Part model, mm, in its own coordinate system. A direction names the side the tool comes from. Give positions to 0.01 mm unless a question says otherwise; leave off trailing zeros. Order: outer loops, then holes, each group sorted by start corner. A loop starts at its lowest first (then second) coordinate and runs counter-clockwise, first axis right, second up. Notation, with made-up numbers: M -23.75,67 L 33.25,67 A35 cw 33.25,100 Z; hole C 22,51 d8. An arc over 180 degrees is marked long. Answer as a JSON object with one key per item and string values.
from build123d import *

# Parameters (mm, degrees)
F1_DEPTH = 10
F2_R     = 5
F3_R     = 2.5
F4_R     = 1.5
F5_DEPTH = 25


with BuildPart() as f1:
    # F0 (on Front) → F1 (new body)
    with BuildSketch(Plane.XZ):
        Polygon((-40.5, 0), (0, 0), (0, -6.2), (7, -6.2), (7, 7.8), (-123, 22.8), (-143, 22.8), (-143, 12.8), (-118, 12.8), (-40.5, -13.2), (-34.5, -13.2), (-34.5, -6.2), (-40.5, -6.2), align=None)
    extrude(amount=F1_DEPTH)

    # F2
    f2_edges = [f1.edges().sort_by_distance(p)[0] for p in [
        (7, -5, 7.8),
    ]]
    fillet(f2_edges, radius=F2_R)

    # F3
    f3_edges = [f1.edges().sort_by_distance(p)[0] for p in [
        (-34.5, -5, -13.2),
        (-40.5, -5, -13.2),
    ]]
    fillet(f3_edges, radius=F3_R)

    # F4 (on face) → F5 (cut)
    with BuildSketch(Plane.XY.offset(22.8)):
        with Locations((-128, -5)):
            Circle(F4_R)
        with Locations((-138, -5)):
            Circle(F4_R)
    extrude(amount=-F5_DEPTH, mode=Mode.SUBTRACT)


solid = f1.part
1. Which spindle directions (+Z, -Z, +X, -X, +Y, -Y) get a long thin tool onto all of the face, cutting with end or side? Do faces 1 (the flat face through (0, -5, -3)), 2 (the flat face through (-131, -5, 12.8)), 3 (the flat face through (-34.5, -5, -8)). Say none if no direction does.
Worked answers:
{"face 1": "-Z, +Y, -Y", "face 2": "-Z, -X, +Y, -Y", "face 3": "-Z, +X, +Y, -Y"}
2. Pin check, flat tips, straight feed: P1, Ø3.5, axis at x = 3.5, y = -5, coming from the -Z side; P2, Ø1.8, axis at x = -39, y = -3, coming from the +Z side; P3, Ø5, axis at y = -6, z = -9, coming from the +X side; P4, Ø2.5, axis at x = -138, y = -5, coming from the -Z side. Stop position of each tip, or through.
Worked answers:
{"P1": "stops at z = -6.2", "P2": "stops at z = 13.21", "P3": "stops at x = -34.5", "P4": "passes through"}
3. Cut at B-B on y = -5. Give the cut face in (x, z).
Worked answers:
{"outline": "M -143,12.8 L -139.5,12.8 L -139.5,22.8 L -143,22.8 Z; M -136.5,12.8 L -129.5,12.8 L -129.5,22.8 L -136.5,22.8 Z; M -126.5,12.8 L -118,12.8 L -40.89,-13.07 A2.5 ccw -40.09,-13.2 L -37,-13.2 A2.5 ccw -34.5,-10.7 L -34.5,-6.2 L -40.5,-6.2 L -40.5,0 L 0,0 L 0,-6.2 L 7,-6.2 L 7,3.34 A5 ccw 2.57,8.31 L -123,22.8 L -126.5,22.8 Z"}
4. Two-plate mould, pull along X, no slides. Class faces 4 (the flat face through (-79.983, -4.93, 0.046)), 5 (the flat face through (-133, -5, 22.8)), 6 (the cylindrical face through (-139.5, -4.93, 17.87)): +X half, -X half, draft (parallel to the pull), parting line (faces both ways), or undercut.
Worked answers:
{"face 4": "-X half", "face 5": "draft", "face 6": "undercut"}
5. Probe line 1 along Y through (x, z) = (-138, 19); line 2 along Z through (x, y) = (-126.5, -2); line 3 along Z through (x, y) = (-52.5, -5.5). List the from-to ranges inside material, lowest first.
Worked answers:
{"line 1": "y = -10 to -6.5, -3.5 to 0", "line 2": "z = 12.8 to 22.8", "line 3": "z = -9.17 to 14.67"}
6. Cut at C-C on z = 18. Give the cut face in (x, y), plus the area to 3 significant figures.
Worked answers:
{"outline": "M -143,-10 L -81.4,-10 L -81.4,0 L -143,0 Z; hole C -138,-5 d3; hole C -128,-5 d3", "area": "602 mm^2"}
7. Cut at D-D on z = -2. Give the cut face in (x, y).
Worked answers:
{"outline": "M -73.88,-10 L -40.5,-10 L -40.5,0 L -73.88,0 Z; M 0,-10 L 7,-10 L 7,0 L 0,0 Z"}
8. Cut at A-A on x = -38.5. Give the cut face in (y, z), plus the area to 4 significant figures.
Worked answers:
{"outline": "M -10,-13.2 L 0,-13.2 L 0,-6.2 L -10,-6.2 Z; M -10,0 L 0,0 L 0,13.05 L -10,13.05 Z", "area": "200.5 mm^2"}
